Could you check a few things on this model? Use its own coordinates, in mm. Round coordinates to 2 decimals unless told otherwise and drop trailing zeros. Loops run counter-clockwise (first coordinate to the right, second up) from the corner with the lowest first, then second, coordinate; pieces in that order, holes last. Notation, with made-up numbers: (61.5, -11.75) -> (85.5, -11.75) arc R28 ccw to (85.5, 11.25) -> close; hole circle Ø2 at (50.25, 62.25). An arc over 180 degrees is marked (long way). Put each result on its own line as item: value. Start each with the question number.
1. Imagine slicing it at B-B, the plane z = 4. Please give me the cut outline in (x, y), and give its area (3 significant figures).
2. Imagine slicing it at C-C, the plane y = -14.5. Please give me the cut outline in (x, z), and give its area (3 significant figures).
3. I need wall thicknesses on line 1 (Z direction, x = 26, y = 11); line 2 (Z direction, x = 3.5, y = -1). Which ranges of each line are inside material? Lowest first, please. Write a range as [from, to].
4. I'm going to push flat-ended pins straight in: P1, Ø4, axis at x = -16, y = -8, coming from the +Z side; P2, Ø6, axis at x = 10.5, y = -4.5, coming from the -Z side; P3, Ø10, axis at x = -13, y = 16.5, coming from the +Z side. Where does each tip first touch, or does it pass through?
```python
from build123d import *

# Parameters (mm, degrees)
F0_W       = 64
F0_H       = 44
F1_DEPTH   = 8
F2_SIZE2   = 21.99999
F2_SIZE    = 7.99999
F2_2_SIZE2 = 21.99999
F2_2_SIZE  = 7.99999


# Not quite as in the source:
# - a fillet or chamfer is up to 0.001 mm smaller than in the source, because OpenCascade refuses the exact size


with BuildPart() as f1:
    # F0 (on Top) → F1 (new body)
    with BuildSketch(Plane.XY):
        Rectangle(F0_W, F0_H)
    extrude(amount=F1_DEPTH)

    # F2 (size 8 and 22 in the source; OpenCascade refuses exactly that, so slightly less here)
    f2_edges = [f1.edges().sort_by_distance(p)[0] for p in [
        (0, -22, 8),
    ]]
    f2_side = f1.faces().sort_by_distance((0, -22, 4))[0]
    chamfer(f2_edges, length=F2_SIZE, length2=F2_SIZE2, reference=f2_side)

    # F2#2 (size 8 and 22 in the source; OpenCascade refuses exactly that, so slightly less here)
    f2_2_edges = [f1.edges().sort_by_distance(p)[0] for p in [
        (0, 22, 8),
    ]]
    f2_2_side = f1.faces().sort_by_distance((0, 22, 4))[0]
    chamfer(f2_2_edges, length=F2_2_SIZE, length2=F2_2_SIZE2, reference=f2_2_side)


solid = f1.part
```
Entries:
1. outline: (-32, -11) -> (32, -11) -> (32, 11) -> (-32, 11) -> close
1. area: 1,410 mm^2
2. outline: (-32, 0) -> (32, 0) -> (32, 2.73) -> (-32, 2.73) -> close
2. area: 175 mm^2
3. line 1: [0, 4]
3. line 2: [0, 7.64]
4. P1: z = 5.82
4. P2: z = 0
4. P3: z = 3.82
